Autodesk Inventor part; units mm, degrees
ref_plane "Arbeitsebene1" through (0, 21, 0) normal (0, 1, 0) x (-1, 0, 0)
ref_plane "YZ Plane" through (0, 0, 0) normal (1, 0, 0) x (0, 1, 0)
ref_plane "XY Plane" through (0, 0, 0) normal (0, 0, 1) x (1, 0, 0)
sketch "Skizze1" plane through (0, 0, 0) normal (0, 0, 1) x (1, 0, 0)
  line L0 (-29.4, 0) -> (29.4, 0)
  line L1 (0, -29.4) -> (0, 29.4)
  circle A0 centre (0, 0) radius 21
  circle A1 centre (0, 0) radius 19.5
  dimension "d0" = 42
  dimension "d1" = 39
extrude "Extrusion1" add sketch "Skizze1" along normal blind 40 contours A1 L1 A0 L0 | L0 A0 L1 A1 | A1 L0 A0 L1 | L1 A0 L0 A1
sketch "Skizze2" plane through (0, 0, 40) normal (0, 0, 1) x (1, 0, 0)
  circle A0 centre (0, 0) radius 19.5
extrude "Extrusion2" add sketch "Skizze2" against normal blind 1
sketch "Skizze3" plane through (0, 0, 40) normal (0, 0, 1) x (1, 0, 0)
  circle A0 centre (0, 0) radius 21
extrude "Extrusion3" add sketch "Skizze3" along normal blind 4
sketch "Skizze4" plane through (0, 0, 0) normal (0, 1, 0) x (-1, 0, 0)
  line L0 (21, 44) -> (-21, 44)
  line L1 (10, 50) -> (-10, 50)
  line L2 (0, -9.2) -> (0, 55.2)
  line L3 (29.4, 0) -> (-29.4, 0)
  line L4 (-10, 50) -> (-6.5359, 44)
  line L5 (10, 50) -> (6.5359, 44)
  line L6 (-6.5359, 44) -> (6.5359, 44)
  point P0 (0, 0)
  dimension "d8" = 20
  dimension "d9" = 6
  dimension "d10" = 60
extrude "Extrusion4" add sketch "Skizze4" along normal mid plane 25
ref_plane "Arbeitsebene1" through (0, 21, 0) normal (0, 1, 0) x (-1, 0, 0)
sketch "Skizze5" plane through (0, 21, 0) normal (0, 1, 0) x (-1, 0, 0)
  line L0 (29.4, 0) -> (-29.4, 0)
  line L1 (0, -10) -> (0, 60)
  point P0 (0, 0)
  point P1 (0, 2)
  dimension "d16" = 2
hole "Bohrung1" at (0, 21, 2) direction (0, -1, 0) diameter 2.4 end through all
pattern_circular "Runde Anordnung1" count 4 over 360 about axis through (0, 0, 0) along (0, 0, 1) of "Bohrung1"
sketch "Skizze6" plane through (-10, 12.5, 50) normal (0, 0, 1) x (1, 0, 0)
  line L0 (0, 0) -> (20, 0)
  line L1 (-19.4018, -12.5) -> (39.4018, -12.5)
  line L2 (10, -41.9018) -> (10, 16.9018)
  circle A0 centre (10, -2.5) radius 1.5
  line L3 (8.5, -2.5) -> (8.5, 0)
  line L4 (11.5, -2.5) -> (11.5, 0)
  line L5 (11.5, 0) -> (8.5, 0)
  point P0 (10, -12.5)
  dimension "d27" = 10
  dimension "d28" = 3
extrude "Extrusion5" cut sketch "Skizze6" against normal up to surface (6 mm away)
chamfer "Fase2" distance 2 angle 45 1 edges at (-21, 0, 44)
sketch "Skizze8" plane through (0, 0, 0) normal (0, 0, -1) x (-1, 0, 0)
  circle A0 centre (0, 0) radius 19.5
  circle A1 centre (0, 0) radius 21
extrude "Extrusion6" cut sketch "Skizze8" against normal up to surface (39 mm away)
sketch "Skizze9" plane through (0, 0, 39) normal (0, 0, -1) x (-1, 0, 0)
  circle A0 centre (0, 0) radius 21
hole "Bohrung2" at (0, 0, 39) direction (0, 0, 1) diameter 4.459 depth 8 tip angle 118
sketch "Skizze11" plane through (0, 0, 39) normal (0, 0, -1) x (-1, 0, 0)
  circle A0 centre (0, 0) radius 21
  circle A1 centre (0, 0) radius 7.5
  line L0 (29.4, 0) -> (-29.4, 0)
  line L1 (0, -29.4) -> (0, 29.4)
  point P0 (-7.5, 0)
  point P1 (7.5, 0)
  dimension "d44" = 15
hole "Bohrung3" at (7.5, 0, 39) at (-7.5, 0, 39) direction (0, 0, 1) diameter 1.567 depth 4 tip angle 118
properties part number "13_1087_061"
Input: part model. Units: mm. Frame: model coordinates. A direction names the side the tool comes from. Round coordinates to 2 decimals unless told otherwise and drop trailing zeros. Loops run counter-clockwise (first coordinate to the right, second up) from the corner with the lowest first, then second, coordinate; pieces in that order, holes last. Notation, with made-up numbers: (-35.75, 56.5) -> (-17.75, 56.5) arc R24 cw to (-17.75, 77.5) -> close; hole circle Ø10 at (50, 40). An arc over 180 degrees is marked (long way). Use one line per item in the form item = value. Start each with the question number.
Item 1: Material intervals for L1, parallel to Y at x = 0, z = 41.25; L2, parallel to Z at x = 12, y = 11.5; L3, parallel to Y at x = 7.5, z = 40.3, sorted ascending. Write a range as from..to.
Item 2: Mould query, pull axis X, two halves, no side actions, for faces 4 (the face through (1.5, 11, 47)), 5 (the face through (8.29, -0.18, 47.04)), 6 (the face through (0, 0, 50)). Classes: pulls with the +X half, pulls with the -X half, needs draft (parallel to the pull), parting line crosses it, or undercut.
Item 3: Contact query for flat-ended pins moving along their axis: pin 1 Ø3 at (y, z) = (12.5, 40.5) entering from +X; pin 2 Ø6.5 at (x, z) = (-7, 48.5) entering from +Y; pin 3 Ø2 at (y, z) = (6, 41.5) entering from +X. Output: stop coordinate, or through.
Item 4: Set-up query: faces 1 (the face through (8.265, -0.17, 41.028)), 2 (the face through (-1.5, 11, 47)), 3 (the face through (0, -12.5, 47)). Return all of +Z, -Z, +X, -X, +Y, -Y with unobstructed straight access to the full face (end or side cutting, diameter ignored); none if empty.
Item 5: Section query A-A on z = 46.5. Return the cut outline in (x, y), then the cut area to 3 significant figures.
Ans:
q1.L1 = -21..-2.23, 2.23..21
q1.L2 = 39..44
q1.L3 = -19.62..-0.78, 0.78..19.62
q2.face_4 = undercut
q2.face_5 = pulls with the +X half
q2.face_6 = needs draft
q3.pin_1 = 17.89
q3.pin_2 = 12.5
q3.pin_3 = 20.4
q4.face_1 = -Z
q4.face_2 = +Z, +Y
q4.face_3 = +Z, +X, -X, -Y
q5.outline = (-7.98, -12.5) -> (7.98, -12.5) -> (7.98, 12.5) -> (1.5, 12.5) -> (1.5, 10) arc R1.5 cw to (-1.5, 10) -> (-1.5, 12.5) -> (-7.98, 12.5) -> close; hole circle Ø4.46 at (0, 0)
q5.area = 372 mm^2
